Read the model definition and answer for the solid it produces. Units are mm, in the model's axes. A direction names the side the tool comes from. Coordinates: 2 decimals unless noted, no trailing zeros. Use a Markdown table: item, result.
from build123d import *

# Parameters (mm, degrees)
SKETCH1_R           = 3
SKETCH1_W           = 15
SKETCH1_H           = 15
BOSS_EXTRUDE1_DEPTH = 5
SKETCH2_R           = 1.5
CUT_EXTRUDE1_DEPTH  = 185
SKETCH3_R           = 2
CUT_EXTRUDE2_DEPTH  = 10


with BuildPart() as part:
    # Sketch1 → Boss-Extrude1 (new body)
    with BuildSketch(Plane.XY):
        Polygon((191.25, 71.637645579), (255, 71.637645579), (255, 0), (191.25, 0), (191.25, -5), (127.5, -5), (63.75, -5), (63.75, 0), (0, 0), (0, 71.637645579), (63.75, 71.637645579), (63.75, 76.637645579), (127.5, 76.637645579), (191.25, 76.637645579), align=None)
        with Locations((81.6684273, 63.35852795)):
            Circle(SKETCH1_R, mode=Mode.SUBTRACT)
        with Locations((173.3315727, 63.35852795)):
            Circle(SKETCH1_R, mode=Mode.SUBTRACT)
        with Locations((81.6684273, 8.27911763)):
            Circle(SKETCH1_R, mode=Mode.SUBTRACT)
        with Locations((173.3315727, 8.27911763)):
            Circle(SKETCH1_R, mode=Mode.SUBTRACT)
        with Locations((127.870410973, 62.57941032)):
            Rectangle(SKETCH1_W, SKETCH1_H, mode=Mode.SUBTRACT)
        with Locations((127.870410973, 9.058235259)):
            Rectangle(SKETCH1_W, SKETCH1_H, mode=Mode.SUBTRACT)
    extrude(amount=BOSS_EXTRUDE1_DEPTH)

    # Sketch2 → Cut-Extrude1 (cut)
    with BuildSketch(Plane(origin=(0, 0, 0), x_dir=(-1, 0, 0), z_dir=(0, 0, -1))):
        with Locations((-31.875, 5)):
            Circle(SKETCH2_R)
        with Locations((-31.875, 66.637645579)):
            Circle(SKETCH2_R)
        with Locations((-223.125, 66.637645579)):
            Circle(SKETCH2_R)
        with Locations((-223.125, 5)):
            Circle(SKETCH2_R)
    extrude(amount=-CUT_EXTRUDE1_DEPTH, mode=Mode.SUBTRACT)

    # Sketch3 → Cut-Extrude2 (cut)
    with BuildSketch(Plane(origin=(0, 0, 0), x_dir=(-1, 0, 0), z_dir=(0, 0, -1))):
        with Locations((-31.875, 5)):
            Circle(SKETCH3_R)
        with Locations((-31.875, 66.637645579)):
            Circle(SKETCH3_R)
        with Locations((-223.125, 5)):
            Circle(SKETCH3_R)
        with Locations((-223.125, 66.637645579)):
            Circle(SKETCH3_R)
    extrude(amount=-CUT_EXTRUDE2_DEPTH, mode=Mode.SUBTRACT)


solid = part.part
(1) Each of these flat-tipped pins is pushed along its axis until it touches: P1, Ø3, axis at x = 223.12, y = 66.64, coming from the +Z side; P2, Ø1.5, axis at y = -1.5, z = 2.5, coming from the -X side; P3, Ø1.5, axis at x = 230.5, z = 2, coming from the -Y side. Where does it stop, or does it pass through?
Report:
| item | result |
|---|---|
| P1 | passes through |
| P2 | stops at x = 63.75 |
| P3 | stops at y = 0 |
(2) Straight lines are drawn through the part: L1, parallel to Y at x = 81.5, z = 1.5; L2, parallel to Y at x = 122, z = 1.9; L3, parallel to X at y = 10, z = 1.3. For each, find the intervals that lie inside material, in ascending order.
Report:
| item | result |
|---|---|
| L1 | y = -5 to 5.28, 11.27 to 60.36, 66.35 to 76.64 |
| L2 | y = -5 to 1.56, 16.56 to 55.08, 70.08 to 76.64 |
| L3 | x = 0 to 79.21, 84.13 to 120.37, 135.37 to 170.87, 175.79 to 255 |
(3) A cutting plane is placed at A-A, the plane z = 3.1. Count the separate pieces of the cut face and the enclosed holes in it, and give its area (3 significant figures).
Report:
| item | result |
|---|---|
| separate pieces | 1 |
| enclosed holes | 10 |
| area | 18,900 mm² |
(4) The mould has two halves that part along Y. Classify faces 1 (the cylindrical face through (176.193, 9.18, 2.465)), 2 (the flat face through (31, 71.638, 2)), 3 (the flat face through (63.75, -3, 2)), 4 (the cylindrical face through (81.278, 66.333, 2.465)): pulls with the +Y half, pulls with the -Y half, needs draft (parallel to the pull), parting line crosses it, or undercut.
Report:
| item | result |
|---|---|
| face 1 | undercut |
| face 2 | pulls with the +Y half |
| face 3 | needs draft |
| face 4 | undercut |
(5) For faces 5 (the flat face through (120.37, 9, 2)), 6 (the flat face through (63.75, 74, 2)), 7 (the flat face through (255, 36, 2)), 8 (the flat face through (223, 71.638, 2)), 9 (the flat face through (224, 0, 2)), determine the directions among +Z, -Z, +X, -X, +Y, -Y from which every point of the face is accessible in a straight line to the end or side of a thin tool.
Report:
| item | result |
|---|---|
| face 5 | +Z, -Z |
| face 6 | +Z, -Z, -X, +Y |
| face 7 | +Z, -Z, +X, +Y, -Y |
| face 8 | +Z, -Z, +X, +Y |
| face 9 | +Z, -Z, +X, -Y |
